Print and shaded views of the part. All mm, measured from the part's lowest x, y and z. A direction names the side the tool comes from. Give positions to 0.01 mm unless a question says otherwise; leave off trailing zeros. Loops run counter-clockwise (first coordinate to the right, second up) from the corner with the lowest first, then second, coordinate; pieces in that order, holes last. Notation, with made-up numbers: M 25.25,-6.5 L 47.25,-6.5 A25 ccw 47.25,21.5 Z; hole C 30.25,24 d9. An arc over 180 degrees is marked long. Put each result on its own line as item: value. Start each with the question number.
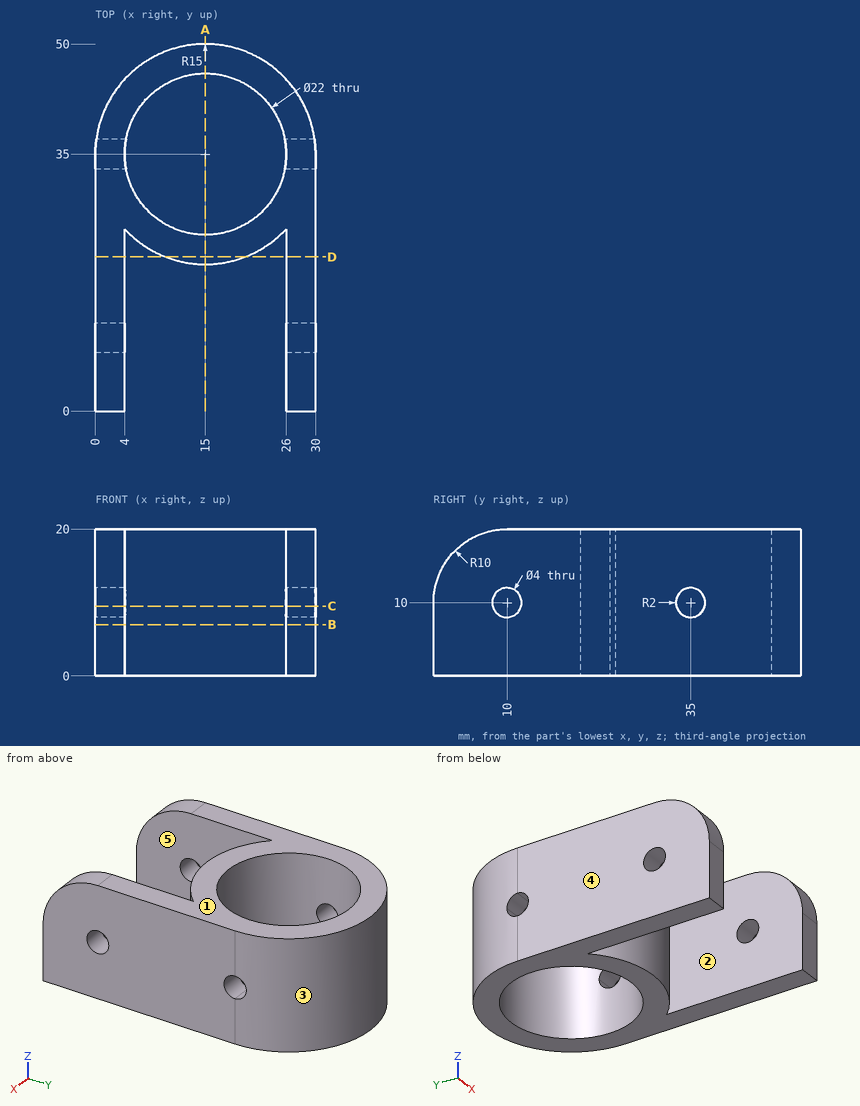
1) Band-saw the part on D-D on y = 21. Give the cut face in (x, z), then the cut area to 3 significant figures.
2) Which spindle directions (+Z, -Z, +X, -X, +Y, -Y) get a long thin tool onto all of the face, cutting with end or side? Do the marked faces 4 and 5. Say none if no direction does.
3) Band-saw the part on A-A on x = 15. Give the cut face in (y, z).
4) Mould opens along X. For the marked faces 1, 2 and 3 say: +X half, -X half, draft (parallel to the pull), parting line (faces both ways), or undercut.
5) Pin check, flat tips, straight feed: pin 1 Ø4 at (y, z) = (44.5, 3.5) entering from +X; pin 2 Ø12 at (x, z) = (18.5, 2.5) entering from -Y. Stop position of each tip, or through.
6) Wall check: L1, parallel to Y at x = 15, z = 16.25; L2, parallel to Z at x = 1, y = 10; L3, parallel to X at y = 35, z = 7.25. Give the ranges that are in metal, low to high.
7) Band-saw the part on C-C on z = 9.5. Give the cut face in (x, y).
8) Band-saw the part on B-B on z = 7. Give the cut face in (x, y), then the cut area to 3 significant figures.
Evaluation:
1. outline: M 0,0 L 4,0 L 4,20 L 0,20 Z; M 9.61,0 L 20.39,0 L 20.39,20 L 9.61,20 Z; M 26,0 L 30,0 L 30,20 L 26,20 Z
1. area: 375 mm2
2. face 4: +Z, -Z, -X, +Y, -Y
2. face 5: +Z, -Z, -Y
3. outline: M 20,0 L 24,0 L 24,20 L 20,20 Z; M 46,0 L 50,0 L 50,20 L 46,20 Z
4. face 1: draft
4. face 2: undercut
4. face 3: parting line
5. pin 1: x = 27.99
5. pin 2: y = 20
6. L1: 20 to 24, 46 to 50
6. L2: 0 to 8, 12 to 20
6. L3: 0 to 4, 26 to 30
7. outline: M 0,0 L 4,0 L 4,8.06 L 0,8.06 Z; M 0,11.94 L 4,11.94 L 4,24.8 A15 ccw 26,24.8 L 26,11.94 L 30,11.94 L 30,33.06 L 25.83,33.06 A11 cw 4.17,33.06 L 0,33.06 Z; M 0.13,36.94 L 4.17,36.94 A11 cw 25.83,36.94 L 29.87,36.94 A15 ccw Z; M 26,0 L 30,0 L 30,8.06 L 26,8.06 Z
8. outline: M 0,0 L 4,0 L 4,24.8 A15 ccw 26,24.8 L 26,0 L 30,0 L 30,35 A15 ccw 0,35 Z; hole C 15,35 d22
8. area: 551 mm2
